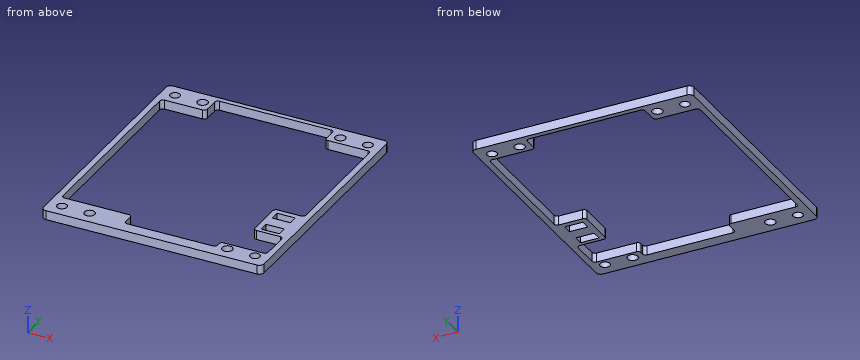
from build123d import *

# Parameters (mm, degrees)
MODEL_R                 = 1.7
MODEL_R_2               = 1.600279216
MODEL_W                 = 6
MODEL_H                 = 3.1
SALIENTE_EXTRUIR1_DEPTH = 3


with BuildPart() as part:
    # Model → Saliente-Extruir1 (new body)
    with BuildSketch(Plane.XY):
        with BuildLine():
            Line((76.985222791, 300.245724916), (7.982818557, 300.245724916))
            ThreePointArc((7.982818557, 300.245724916), (6.922158385, 299.806385087), (6.482818557, 298.745724916))
            Line((6.482818557, 298.745724916), (6.482818557, 220.741115058))
            ThreePointArc((6.482818557, 220.741115058), (6.922158385, 219.680454886), (7.982818557, 219.241115058))
            Line((7.982818557, 219.241115058), (76.985222791, 219.241115058))
            ThreePointArc((76.985222791, 219.241115058), (78.045882963, 219.680454886), (78.485222791, 220.741115058))
            Line((78.485222791, 220.741115058), (78.485222791, 298.745724916))
            ThreePointArc((78.485222791, 298.745724916), (78.045882963, 299.806385087), (76.985222791, 300.245724916))
        make_face()
        with Locations((19.982149553, 223.740780556)):
            Circle(MODEL_R, mode=Mode.SUBTRACT)
        with Locations((64.985557294, 223.740780556)):
            Circle(MODEL_R, mode=Mode.SUBTRACT)
        with Locations((10.982484055, 223.740780556)):
            Circle(MODEL_R_2, mode=Mode.SUBTRACT)
        with Locations((73.985222791, 223.740780556)):
            Circle(MODEL_R_2, mode=Mode.SUBTRACT)
        with Locations((19.982149553, 295.745724916)):
            Circle(MODEL_R, mode=Mode.SUBTRACT)
        with Locations((64.985557294, 295.745724916)):
            Circle(MODEL_R, mode=Mode.SUBTRACT)
        with Locations((73.985222791, 295.745724916)):
            Circle(MODEL_R_2, mode=Mode.SUBTRACT)
        with Locations((10.982484055, 295.745724916)):
            Circle(MODEL_R_2, mode=Mode.SUBTRACT)
        with BuildLine():
            Line((76.48504158, 291.747923326), (76.48504158, 251.338841953))
            ThreePointArc((76.48504158, 251.338841953), (76.192148361, 250.631735172), (75.48504158, 250.338841953))
            Line((75.48504158, 250.338841953), (67.705071812, 250.338841953))
            ThreePointArc((67.705071812, 250.338841953), (66.997954371, 250.045938075), (66.705071812, 249.338811805))
            Line((66.705071812, 249.338811805), (66.705414934, 237.957679154))
            ThreePointArc((66.705414934, 237.957679154), (66.998318811, 237.250591862), (67.705414933, 236.957709302))
            Line((67.705414933, 236.957709302), (75.48504158, 236.957709302))
            ThreePointArc((75.48504158, 236.957709302), (76.192148361, 236.664816083), (76.48504158, 235.957709302))
            Line((76.48504158, 235.957709302), (76.48504158, 227.243313469))
            ThreePointArc((76.48504158, 227.243313469), (76.192148361, 226.536206687), (75.48504158, 226.243313469))
            Line((75.48504158, 226.243313469), (62.48504158, 226.243313469))
            ThreePointArc((62.48504158, 226.243313469), (61.777934798, 225.95042025), (61.48504158, 225.243313469))
            Line((61.48504158, 225.243313469), (61.48504158, 224.241115058))
            ThreePointArc((61.48504158, 224.241115058), (61.192148361, 223.534008277), (60.48504158, 223.241115058))
            Line((60.48504158, 223.241115058), (32.482637345, 223.241115058))
            ThreePointArc((32.482637345, 223.241115058), (31.775530564, 223.534008277), (31.482637345, 224.241115058))
            Line((31.482637345, 224.241115058), (31.482637345, 227.21772226))
            ThreePointArc((31.482637345, 227.21772226), (31.189744126, 227.924829041), (30.482637345, 228.21772226))
            Line((30.482637345, 228.21772226), (9.482637345, 228.21772226))
            ThreePointArc((9.482637345, 228.21772226), (8.775530564, 228.510615479), (8.482637345, 229.21772226))
            Line((8.482637345, 229.21772226), (8.482637345, 290.857923326))
            ThreePointArc((8.482637345, 290.857923326), (8.775530564, 291.565030108), (9.482637345, 291.857923326))
            Line((9.482637345, 291.857923326), (21.982637345, 291.857923326))
            ThreePointArc((21.982637345, 291.857923326), (22.689744126, 292.150816545), (22.982637345, 292.857923326))
            Line((22.982637345, 292.857923326), (22.982637345, 297.584751174))
            ThreePointArc((22.982637345, 297.584751174), (23.275530564, 298.291857955), (23.982637345, 298.584751174))
            Line((23.982637345, 298.584751174), (60.48504158, 298.584751174))
            ThreePointArc((60.48504158, 298.584751174), (61.192148361, 298.291857955), (61.48504158, 297.584751174))
            Line((61.48504158, 297.584751174), (61.48504158, 293.747923326))
            ThreePointArc((61.48504158, 293.747923326), (61.777934798, 293.040816545), (62.48504158, 292.747923326))
            Line((62.48504158, 292.747923326), (75.48504158, 292.747923326))
            ThreePointArc((75.48504158, 292.747923326), (76.192148361, 292.455030108), (76.48504158, 291.747923326))
        make_face(mode=Mode.SUBTRACT)
        with Locations((71.494936084, 246.999441896)):
            Rectangle(MODEL_W, MODEL_H, mode=Mode.SUBTRACT)
        with Locations((71.494936084, 239.854068189)):
            Rectangle(MODEL_W, MODEL_H, mode=Mode.SUBTRACT)
    extrude(amount=SALIENTE_EXTRUIR1_DEPTH)


solid = part.part
The listing builds one solid part. Answer for the finished solid, in the listing's coordinates (mm). Round coordinates to 2 decimals unless told otherwise and drop trailing zeros. Loops run counter-clockwise (first coordinate to the right, second up) from the corner with the lowest first, then second, coordinate; pieces in that order, holes last. Notation, with made-up numbers: M -29.5,-15.5 L 25.5,-15.5 A5 cw 25.5,-6.5 Z; hole C 23,12 d9. An arc over 180 degrees is marked long. Return JSON: item names as keys, results as strings.
Q1. Find section A-A, the plane y = 263.5. Determine the outline of the cut face in (x, z).
Results list:
{"outline": "M 6.48,0 L 8.48,0 L 8.48,3 L 6.48,3 Z; M 76.49,0 L 78.49,0 L 78.49,3 L 76.49,3 Z"}
Q2. Each of these flat-tipped pins is pushed along its axis until it touches: pin 1 Ø12 at (x, y) = (65, 272) entering from -Z; pin 2 Ø5 at (x, y) = (10.98, 295.75) entering from +Z. Where does it stop, or does it pass through?
Results list:
{"pin 1": "passes through", "pin 2": "stops at z = 3"}
Q3. Find section C-C, the plane z = 2.05. State how many separate pieces and enclosed holes the cut face has, plus the area to 3 significant figures.
Results list:
{"separate pieces": "1", "enclosed holes": "11", "area": "1,080 mm2"}
Q4. Find section B-B, the plane x = 17. Determine the outline of the cut face in (y, z).
Results list:
{"outline": "M 219.24,0 L 228.22,0 L 228.22,3 L 219.24,3 Z; M 291.86,0 L 300.25,0 L 300.25,3 L 291.86,3 Z"}
Q5. Find the intervals of material crossed by line 1 along X through (y, z) = (239.5, 1.2); line 2 along X through (y, z) = (265, 2.7); line 3 along Y through (x, z) = (33.5, 0.35), in increasing order. Write a range as from..to.
Results list:
{"line 1": "x = 6.48..8.48, 66.71..68.49, 74.49..78.49", "line 2": "x = 6.48..8.48, 76.49..78.49", "line 3": "y = 219.24..223.24, 298.58..300.25"}
